from build123d import *

# Parameters (mm, degrees)
SKETCH1_R           = 8
BOSS_EXTRUDE1_DEPTH = 4
SKETCH3_R           = 8
BOSS_EXTRUDE3_DEPTH = 4.5
SKETCH2_R           = 0.4
BOSS_EXTRUDE2_DEPTH = 8.5


with BuildPart() as part:
    # Sketch1 → Boss-Extrude1 (new body)
    with BuildSketch(Plane(origin=(0, 0, 0), x_dir=(1, 0, 0), z_dir=(0, 1, 0))):
        Circle(SKETCH1_R)
        Polygon((5.773502692, 0), (2.886751346, 5), (-2.886751346, 5), (-5.773502692, 0), (-2.886751346, -5), (2.886751346, -5), align=None, mode=Mode.SUBTRACT)
    extrude(amount=BOSS_EXTRUDE1_DEPTH)

    # Sketch3 → Boss-Extrude3 (add)
    with BuildSketch(Plane(origin=(0, 4, 0), x_dir=(1, 0, 0), z_dir=(0, 1, 0))):
        Circle(SKETCH3_R)
    extrude(amount=BOSS_EXTRUDE3_DEPTH)

    # Sketch2 → Boss-Extrude2 (add, through all)
    with BuildSketch(Plane(origin=(0, 8.5, 0), x_dir=(1, 0, 0), z_dir=(0, 1, 0))):
        with Locations((0, 7.8)):
            Circle(SKETCH2_R)
        with Locations((1.062099863, 7.727350379)):
            Circle(SKETCH2_R)
        with Locations((2.104414815, 7.510754841)):
            Circle(SKETCH2_R)
        with Locations((3.107528501, 7.154248152)):
            Circle(SKETCH2_R)
        with Locations((4.05275481, 6.664471355)):
            Circle(SKETCH2_R)
        with Locations((4.922485966, 6.050548067)):
            Circle(SKETCH2_R)
        with Locations((5.700520521, 5.323914517)):
            Circle(SKETCH2_R)
        with Locations((6.372365165, 4.498106512)):
            Circle(SKETCH2_R)
        with Locations((6.925504704, 3.588507294)):
            Circle(SKETCH2_R)
        with Locations((7.349635193, 2.612060975)):
            Circle(SKETCH2_R)
        with Locations((7.636855884, 1.586956902)):
            Circle(SKETCH2_R)
        with Locations((7.7818164, 0.532290824)):
            Circle(SKETCH2_R)
        with Locations((7.7818164, -0.532290824)):
            Circle(SKETCH2_R)
        with Locations((7.636855884, -1.586956902)):
            Circle(SKETCH2_R)
        with Locations((7.349635193, -2.612060975)):
            Circle(SKETCH2_R)
        with Locations((6.925504704, -3.588507294)):
            Circle(SKETCH2_R)
        with Locations((6.372365165, -4.498106512)):
            Circle(SKETCH2_R)
        with Locations((5.700520521, -5.323914517)):
            Circle(SKETCH2_R)
        with Locations((4.922485966, -6.050548067)):
            Circle(SKETCH2_R)
        with Locations((4.05275481, -6.664471355)):
            Circle(SKETCH2_R)
        with Locations((3.107528501, -7.154248152)):
            Circle(SKETCH2_R)
        with Locations((2.104414815, -7.510754841)):
            Circle(SKETCH2_R)
        with Locations((1.062099863, -7.727350379)):
            Circle(SKETCH2_R)
        with Locations((0, -7.8)):
            Circle(SKETCH2_R)
        with Locations((-1.062099863, -7.727350379)):
            Circle(SKETCH2_R)
        with Locations((-2.104414815, -7.510754841)):
            Circle(SKETCH2_R)
        with Locations((-3.107528501, -7.154248152)):
            Circle(SKETCH2_R)
        with Locations((-4.05275481, -6.664471355)):
            Circle(SKETCH2_R)
        with Locations((-4.922485966, -6.050548067)):
            Circle(SKETCH2_R)
        with Locations((-5.700520521, -5.323914517)):
            Circle(SKETCH2_R)
        with Locations((-6.372365165, -4.498106512)):
            Circle(SKETCH2_R)
        with Locations((-6.925504704, -3.588507294)):
            Circle(SKETCH2_R)
        with Locations((-7.349635193, -2.612060975)):
            Circle(SKETCH2_R)
        with Locations((-7.636855884, -1.586956902)):
            Circle(SKETCH2_R)
        with Locations((-7.7818164, -0.532290824)):
            Circle(SKETCH2_R)
        with Locations((-7.7818164, 0.532290824)):
            Circle(SKETCH2_R)
        with Locations((-7.636855884, 1.586956902)):
            Circle(SKETCH2_R)
        with Locations((-7.349635193, 2.612060975)):
            Circle(SKETCH2_R)
        with Locations((-6.925504704, 3.588507294)):
            Circle(SKETCH2_R)
        with Locations((-6.372365165, 4.498106512)):
            Circle(SKETCH2_R)
        with Locations((-5.700520521, 5.323914517)):
            Circle(SKETCH2_R)
        with Locations((-4.922485966, 6.050548067)):
            Circle(SKETCH2_R)
        with Locations((-4.05275481, 6.664471355)):
            Circle(SKETCH2_R)
        with Locations((-3.107528501, 7.154248152)):
            Circle(SKETCH2_R)
        with Locations((-2.104414815, 7.510754841)):
            Circle(SKETCH2_R)
        with Locations((-1.062099863, 7.727350379)):
            Circle(SKETCH2_R)
    extrude(amount=-BOSS_EXTRUDE2_DEPTH)


solid = part.part
Read the model definition and answer for the solid it produces. Units are mm, in the model's axes. A direction names the side the tool comes from. Coordinates: 2 decimals unless noted, no trailing zeros. Order: outer loops, then holes, each group sorted by start corner. A loop starts at its lowest first (then second) coordinate and runs counter-clockwise, first axis right, second up. Notation, with made-up numbers: M -32,23 L -17,23 A17 ccw -17,49 Z; hole C 53.25,-26.5 d10. An arc over 180 degrees is marked long. Put each result on its own line as item: value. Start each with the question number.
Item 1: Section B-B, the plane z = -0.5 is taken. Determine the outline of the cut face in (x, y).
Item 2: Given pin 1 Ø1.2 at (x, y) = (-1, 1) entering from +Z; pin 2 Ø1.5 at (y, z) = (7, -6) entering from -X; pin 3 Ø5 at (x, z) = (-0.5, 1) entering from -Y, each flat-ended and moving along its own axis, determine where each tip first touches the part or whether it passes through.
Item 3: The mould has two halves that part along Z. Classify faces 3 (the face through (0, 8.5, 0)), 4 (the face through (0, 2, 5)): +Z half, -Z half, draft (parallel to the pull), parting line (faces both ways), or undercut.
Item 4: For faces 1 (the face through (0, 4, 0)), 2 (the face through (-4, 0, 4)), determine the directions among +Z, -Z, +X, -X, +Y, -Y from which every point of the face is accessible in a straight line to the end or side of a thin tool.
Item 5: Section A-A, the plane x = 2.25 is taken. Determine the outline of the cut face in (y, z).
Item 6: Consider probe 1 along Z at (x, y) = (-1.5, 1.25); probe 2 along Y at (x, z) = (2.5, 3); probe 3 along Z at (x, y) = (0.25, 1.75). Determine where each line is inside the solid, lowest interval first. Write a range as [from, to].
Computed:
1. outline: M -8.18,0 L -5.48,0 L -5.48,4 L 5.48,4 L 5.48,0 L 8.18,0 L 8.18,8.5 L -8.18,8.5 Z
2. pin 1: stops at z = 8.13
2. pin 2: stops at x = -6.1
2. pin 3: stops at y = 4
3. face 3: draft
3. face 4: undercut
4. face 1: -Y
4. face 2: +Z, -Z, +X, -X, -Y
5. outline: M 0,-7.88 L 8.5,-7.88 L 8.5,7.88 L 0,7.88 L 0,5 L 4,5 L 4,-5 L 0,-5 Z
6. probe 1: z = [-7.86, -5], [5, 7.86]
6. probe 2: y = [4, 8.5]
6. probe 3: z = [-8.11, -5], [5, 8.11]
